Build history of the part. All positions in model axes, mm. Face numbers are marked on the shaded views. A direction names the side the tool comes from. Give positions to 0.01 mm unless a question says otherwise; leave off trailing zeros. Use a Markdown table: item, result.
from build123d import *

# Parameters (mm, degrees)
SKETCH1_W           = 30
SKETCH1_H           = 30
BOSS_EXTRUDE1_DEPTH = 80


with BuildPart() as part:
    # Sketch1 → Boss-Extrude1 (new body)
    with BuildSketch(Plane(origin=(0, 0, 0), x_dir=(1, 0, 0), z_dir=(0, 1, 0))):
        with Locations((-27.711864407, 2.161016949)):
            Rectangle(SKETCH1_W, SKETCH1_H)
    extrude(amount=-BOSS_EXTRUDE1_DEPTH)

    # Sketch2 → Revolve4 (revolve)
    with BuildSketch(Plane(origin=(0, 0, -2.161016949), x_dir=(-1, 0, 0), z_dir=(0, 0, -1))):
        with BuildLine():
            Line((27.711864407, 0), (34.551820017, 0))
            ThreePointArc((34.551820017, 0), (31.152183546, 0.559787224), (27.711864407, 0.747121391))
            Line((27.711864407, 0.747121391), (27.711864407, 0))
        make_face()
    revolve(axis=Axis((-27.711864407, -84, -2.161016949), (0, 1, 0)))


solid = part.part
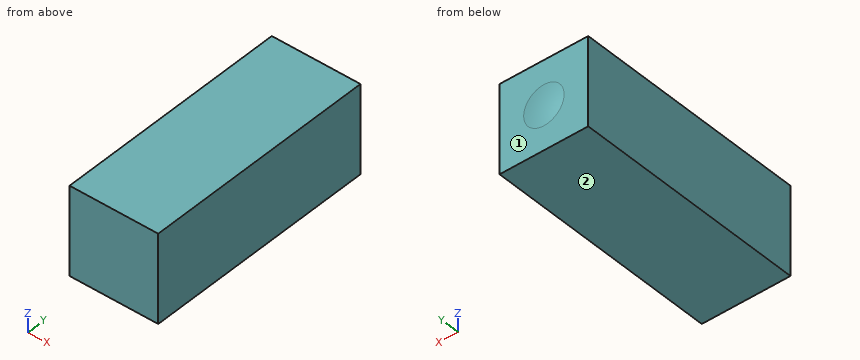
1) Pin check, flat tip, straight feed: P1, Ø5, axis at x = -16.5, z = 2.5, coming from the +Y side. Stop position of the tip, or through.
Computed:
| item | result |
|---|---|
| P1 | stops at y = 0 |
2) Wall check: line 1 (Y direction, x = -30.25, z = -10.75); line 2 (Y direction, x = -23.5, z = 2.5). Give the ranges that are in metal, low to high. Write a range as from..to.
Computed:
| item | result |
|---|---|
| line 1 | y = -80..0 |
| line 2 | y = -80..0.12 |
3) Tool access for the marked faces 1 and 2: list every direction of +Z, -Z, +X, -X, +Y, -Y with a clear straight run to the whole face (end or side of a thin tool).
Computed:
| item | result |
|---|---|
| face 1 | +Y |
| face 2 | -Z, +X, -X, +Y, -Y |
